Design review of the part built by this model. Coordinates are the model's own, in mm. Round coordinates to 2 decimals unless told otherwise and drop trailing zeros. Order: outer loops, then holes, each group sorted by start corner. A loop starts at its lowest first (then second) coordinate and runs counter-clockwise, first axis right, second up. Notation, with made-up numbers: (35.25, 87.25) - (79.25, 87.25) arc R26 cw to (79.25, 106.25) - close; hole circle Ø2 at (78.25, -18). An arc over 180 degrees is marked (long way). Use CSV: the item, a comma, the result in double quotes. Start each with the question number.
from build123d import *

# Parameters (mm, degrees)
SKETCH_1_W          = 10
SKETCH_1_H          = 10
SKETCH_1_W_2        = 8
SKETCH_1_H_2        = 8
EXTRUDE_1_DEPTH     = 120
SKETCH_2_R          = 3
CUT_EXTRUDE_1_DEPTH = 121.519707932
SKETCH_3_R          = 3
CUT_EXTRUDE_2_DEPTH = 10
SKETCH_4_R          = 1.6
CUT_EXTRUDE_3_DEPTH = 10
SKETCH_5_R          = 1.6
CUT_EXTRUDE_4_DEPTH = 121.519707932
SKETCH_6_R          = 3
CUT_EXTRUDE_5_DEPTH = 2


with BuildPart() as part:
    # ｽｹｯﾁ1 → ﾎﾞｽ - 押し出し1 (new body)
    with BuildSketch(Plane.XY):
        Rectangle(SKETCH_1_W, SKETCH_1_H)
        Rectangle(SKETCH_1_W_2, SKETCH_1_H_2, mode=Mode.SUBTRACT)
    extrude(amount=EXTRUDE_1_DEPTH)

    # ｽｹｯﾁ2 → ｶｯﾄ - 押し出し1 (cut, through all)
    with BuildSketch(Plane.ZY.offset(5)):
        with Locations((5, 0)):
            Circle(SKETCH_2_R)
        with Locations((115, 0)):
            Circle(SKETCH_2_R)
    extrude(amount=-CUT_EXTRUDE_1_DEPTH, mode=Mode.SUBTRACT)

    # ｽｹｯﾁ3 → ｶｯﾄ - 押し出し2 (cut)
    with BuildSketch(Plane(origin=(0, 5, 0), x_dir=(1, 0, 0), z_dir=(0, 1, 0))):
        with Locations(Location((0, -105, 0), (0, 0, 270))):
            Circle(SKETCH_3_R)
        with Locations(Location((0, -15, 0), (0, 0, 270))):
            Circle(SKETCH_3_R)
    extrude(amount=-CUT_EXTRUDE_2_DEPTH, mode=Mode.SUBTRACT)

    # ｽｹｯﾁ4 → ｶｯﾄ - 押し出し3 (cut)
    with BuildSketch(Plane(origin=(0, 5, 0), x_dir=(1, 0, 0), z_dir=(0, 1, 0))):
        with Locations(Location((0, -40, 0), (0, 0, 270))):
            Circle(SKETCH_4_R)
        with Locations(Location((0, -80, 0), (0, 0, 270))):
            Circle(SKETCH_4_R)
    extrude(amount=-CUT_EXTRUDE_3_DEPTH, mode=Mode.SUBTRACT)

    # ｽｹｯﾁ5 → ｶｯﾄ - 押し出し4 (cut, through all)
    with BuildSketch(Plane.ZY.offset(5)):
        with Locations((25, 0)):
            Circle(SKETCH_5_R)
        with Locations((95, 0)):
            Circle(SKETCH_5_R)
    extrude(amount=-CUT_EXTRUDE_4_DEPTH, mode=Mode.SUBTRACT)

    # ｽｹｯﾁ6 → ｶｯﾄ - 押し出し5 (cut)
    with BuildSketch(Plane(origin=(0, -5, 0), x_dir=(-1, 0, 0), z_dir=(0, -1, 0))):
        with Locations(Location((0, -40, 0), (0, 0, 90))):
            Circle(SKETCH_6_R)
        with Locations(Location((0, -80, 0), (0, 0, 90))):
            Circle(SKETCH_6_R)
    extrude(amount=-CUT_EXTRUDE_5_DEPTH, mode=Mode.SUBTRACT)


solid = part.part
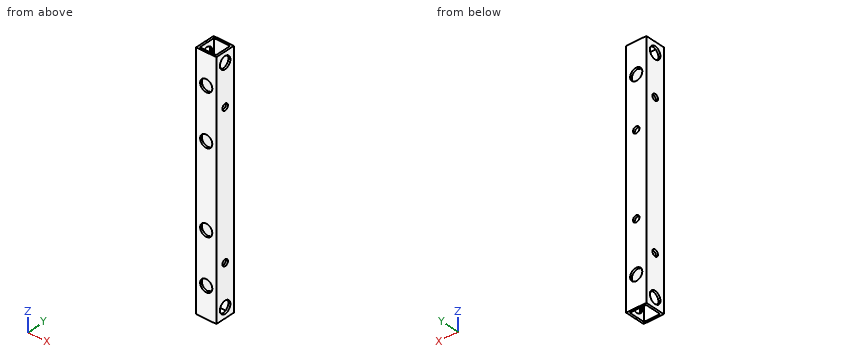
Q1. Take a section at D-D (z = 95). State the section outline as (x, y) points, plus the area to 3 significant figures.
Q2. Take a section at B-B (z = 34). State the section outline as (x, y) points, plus the area to 3 significant figures.
Q3. Clearance check with a flat-ended pin moving along its axis: pin 1 (2.5 mm diameter, centred on y = 0, z = 25, fed in from +X). State where the tip first meets the part, or that it passes through.
Q4. Take a section at C-C (y = 0). Give the number of separate pieces and of enclosed holes in the cut face, plus the area to 3 significant figures.
Q5. Take a section at A-A (z = 5). State the section outline as (x, y) points, plus the area to 3 significant figures.
Q6. For L1, parallel to X at y = -0.5, z = 30; L2, parallel to Z at x = 1, y = 4.5, list the stretches that pass through material, from the lowest coordinate up. Write a range as [from, to].
Findings below:
1,outline,"(-5, -5) - (5, -5) - (5, -1.6) - (4, -1.6) - (4, -4) - (-4, -4) - (-4, -1.6) - (-5, -1.6) - close; (-5, 1.6) - (-4, 1.6) - (-4, 4) - (4, 4) - (4, 1.6) - (5, 1.6) - (5, 5) - (-5, 5) - close"
1,area,"29.6 mm^2"
2,outline,"(-5, -5) - (5, -5) - (5, 5) - (-5, 5) - close; hole (-4, -4) - (4, -4) - (4, 4) - (-4, 4) - close"
2,area,"36.0 mm^2"
3,pin 1,"passes through"
4,separate pieces,"10"
4,enclosed holes,"0"
4,area,"203 mm^2"
5,outline,"(-5, -5) - (5, -5) - (5, -3) - (4, -3) - (4, -4) - (-4, -4) - (-4, -3) - (-5, -3) - close; (-5, 3) - (-4, 3) - (-4, 4) - (4, 4) - (4, 3) - (5, 3) - (5, 5) - (-5, 5) - close"
5,area,"24.0 mm^2"
6,L1,"x = [-5, -4], [4, 5]"
6,L2,"z = [0, 12.17], [17.83, 38.75], [41.25, 78.75], [81.25, 102.17], [107.83, 120]"
